Source: CAD feature listing. Evaluate the final solid. Frame: model axes, mm. A direction names the side the tool comes from. Give positions to 0.01 mm unless a question says otherwise; leave off trailing zeros. Order: outer loops, then holes, each group sorted by start corner. A loop starts at its lowest first (then second) coordinate and runs counter-clockwise, first axis right, second up. Notation, with made-up numbers: M 5,-14 L 12,-14 A31 cw 12,19 Z; hole C -1.75,60 d8. An arc over 180 degrees is marked long. Answer as a JSON object with one key per item and string values. Group by question number.
1. Section query A-A (x = 0). Output: boundary loops of the cut face in (y, z), plus the area to 3 significant figures.
2. Pin query (flat end, axial travel): P1, Ø1.5, axis at x = -14.5, z = 1.5, coming from the -Y side; P2, Ø1.8, axis at x = -15, z = 2.5, coming from the +Y side; P3, Ø4, axis at x = 0, y = 12, coming from the -Z side. Return the tip coordinate at first contact, or that it passes through.
3. Pull-direction query (X, two-part tool) for faces 1 (the flat face through (0, -40, 3)), 2 (the flat face through (5, -1, 3)), 3 (the cylindrical face through (-0.336, 10.487, 2.958)), 4 (the cylindrical face through (0.715, -1.375, 2.958)); classes: +X half, -X half, draft (parallel to the pull), parting line (faces both ways), or undercut.
4. Section query B-B (y = -12). Output: boundary loops of the cut face in (x, z).
5. Set-up query: faces 5 (the flat face through (-5, -22, 3)), 6 (the flat face through (-5, 0, 0)), 7 (the flat face through (-20, 5, 3)). Return all of +Z, -Z, +X, -X, +Y, -Y with unobstructed straight access to the full face (end or side cutting, diameter ignored); none if empty.
6. Material intervals for L1, parallel to Y at x = 0, z = 3.6; L2, parallel to X at y = 9.5, z = 1.9, sorted ascending. Write a range as [from, to].
7. Section query C-C (z = 1.85). Output: boundary loops of the cut face in (x, y).
8. Section query D-D (y = 0). Output: boundary loops of the cut face in (x, z).
from build123d import *

# Parameters (mm, degrees)
SKETCH_1_W      = 10
SKETCH_1_H      = 80
SKETCH_1_R      = 1.55
SKETCH_1_W_2    = 30
SKETCH_1_H_2    = 10
EXTRUDE_1_DEPTH = 6
FILLET_1_R      = 1


with BuildPart() as part:
    # 草图1 → 凸台-拉伸1 (new body)
    with BuildSketch(Plane.XY):
        Rectangle(SKETCH_1_W, SKETCH_1_H)
        with Locations((0, 12)):
            Circle(SKETCH_1_R, mode=Mode.SUBTRACT)
        Circle(SKETCH_1_R, mode=Mode.SUBTRACT)
        with Locations((0, -12)):
            Circle(SKETCH_1_R, mode=Mode.SUBTRACT)
        with Locations((-20, 0)):
            Rectangle(SKETCH_1_W_2, SKETCH_1_H_2)
    extrude(amount=EXTRUDE_1_DEPTH)

    # 圆角1
    fillet_1_edges = [part.edges().sort_by_distance(p)[0] for p in [
        (-5, 40, 3),
        (5, 40, 3),
        (5, -40, 3),
        (-5, -40, 3),
        (-35, -5, 3),
        (-35, 5, 3),
    ]]
    fillet(fillet_1_edges, radius=FILLET_1_R)


solid = part.part
Answer sheet:
{
 "1": {"outline": "M -40,0 L -13.55,0 L -13.55,6 L -40,6 Z; M -10.45,0 L -1.55,0 L -1.55,6 L -10.45,6 Z; M 1.55,0 L 10.45,0 L 10.45,6 L 1.55,6 Z; M 13.55,0 L 40,0 L 40,6 L 13.55,6 Z", "area": "424 mm^2"},
 "2": {"P1": "y = -5", "P2": "y = 5", "P3": "z = 0"},
 "3": {"face 1": "draft", "face 2": "+X half", "face 3": "undercut", "face 4": "undercut"},
 "4": {"outline": "M -5,0 L -1.55,0 L -1.55,6 L -5,6 Z; M 1.55,0 L 5,0 L 5,6 L 1.55,6 Z"},
 "5": {"face 5": "+Z, -Z, -X, -Y", "face 6": "-Z, +X, -X, +Y, -Y", "face 7": "+Z, -Z, -X, +Y"},
 "6": {"L1": "[-40, -13.55], [-10.45, -1.55], [1.55, 10.45], [13.55, 40]", "L2": "[-5, 5]"},
 "7": {"outline": "M -35,-4 A1 ccw -34,-5 L -5,-5 L -5,-39 A1 ccw -4,-40 L 4,-40 A1 ccw 5,-39 L 5,39 A1 ccw 4,40 L -4,40 A1 ccw -5,39 L -5,5 L -34,5 A1 ccw -35,4 Z; hole C 0,-12 d3.1; hole C 0,0 d3.1; hole C 0,12 d3.1"},
 "8": {"outline": "M -35,0 L -1.55,0 L -1.55,6 L -35,6 Z; M 1.55,0 L 5,0 L 5,6 L 1.55,6 Z"}
}
